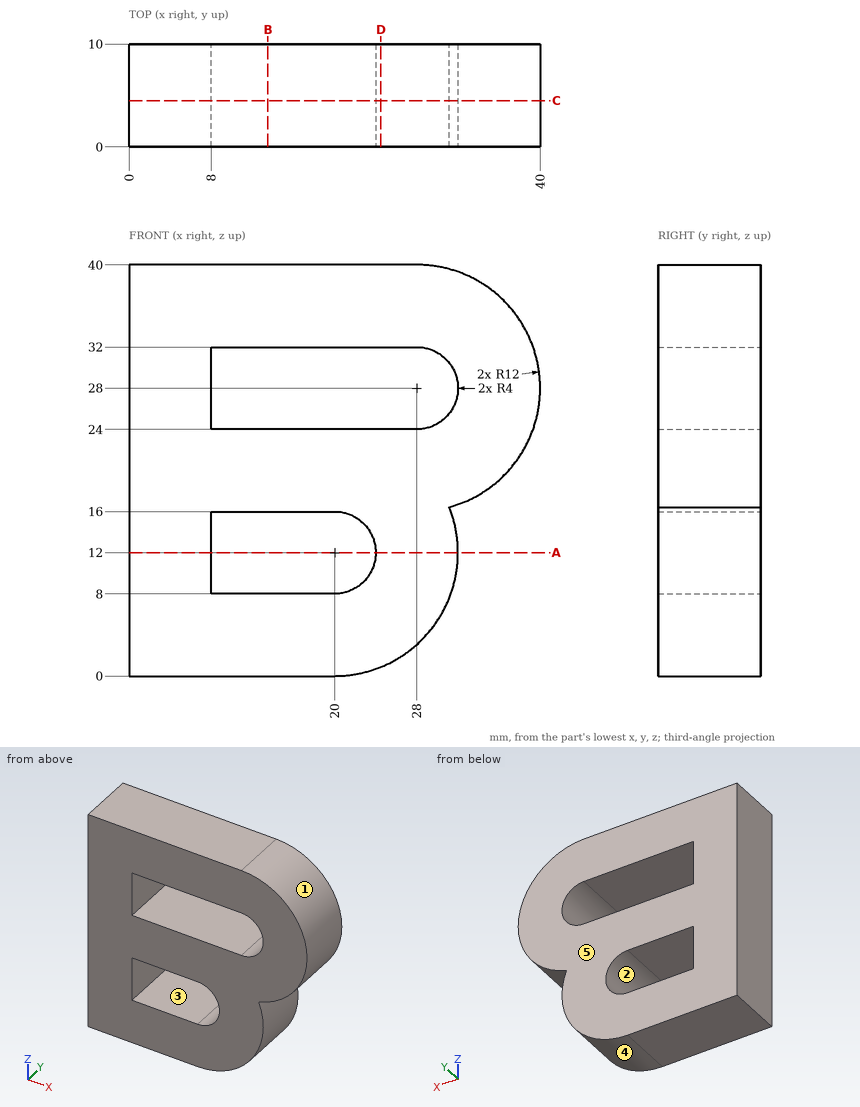
Here's the drawing with two shaded views (mm, measured from the low corner). I have some questions. A direction names the side the tool comes from. Give positions to 0.01 mm unless a question says otherwise; leave off trailing zeros. Write each loop counter-clockwise with the first axis right and the second up, starting at its lowest first coordinate (ties: lowest second). Pieces come first, ordered by that corner, then holes. Notation, with made-up numbers: (87, 60) - (103, 60) arc R27 cw to (103, 85) - close; hole circle Ø5 at (84, -33). An arc over 180 degrees is marked (long way). One line per item, written item: value. Start each with the question number.
Item 1: If we mould it in two halves opening along X, with no side actions, what happens to the marked faces 3, 4 and 5? For each: +X half, -X half, draft (parallel to the pull), parting line (faces both ways), or undercut.
Item 2: Imagine slicing it at C-C, the plane y = 4.5. List the corners of the cut face in (x, z) for me.
Item 3: I'm going to push a flat-ended pin straight in: pin 1 (5 mm diameter, centred on y = 7.5, z = 20.5, fed in from +X). Where does the tip first touch, or does it pass through?
Item 4: Imagine slicing it at A-A, the plane z = 12. List the corners of the cut face in (x, y) for me, and give its area (3 significant figures).
Item 5: Please list where these lines run through material, in increasing order: line 1 (Z direction, x = 17, y = 0.75); line 2 (X direction, y = 7, z = 12.5); line 3 (Z direction, x = 21, y = 8.5). Write a range as from..to.
Item 6: Which directions (+Z, -Z, +X, -X, +Y, -Y) give clear straight access to the entire face, cutting with the end or side of a thin tool? Please do the marked faces 1 and 2.
Item 7: Imagine slicing it at B-B, the plane x = 13.5. List the corners of the cut face in (y, z) for me, and give its area (3 significant figures).
Item 8: Imagine slicing it at D-D, the plane x = 24.5. List the corners of the cut face in (y, z) for me, and give its area (3 significant figures).
Geometry says:
1. face 3: undercut
1. face 4: +X half
1. face 5: draft
2. outline: (0, 0) - (20, 0) arc R12 ccw to (31.16, 16.42) arc R12 ccw to (28, 40) - (0, 40) - close; hole (8, 8) - (20, 8) arc R4 ccw to (20, 16) - (8, 16) - close; hole (8, 24) - (28, 24) arc R4 ccw to (28, 32) - (8, 32) - close
3. pin 1: x = 38.91
4. outline: (0, 0) - (8, 0) - (8, 10) - (0, 10) - close; (24, 0) - (32, 0) - (32, 10) - (24, 10) - close
4. area: 160 mm^2
5. line 1: 0..8, 16..24, 32..40
5. line 2: 0..8, 23.97..31.99
5. line 3: 0.04..8.13, 15.87..24, 32..40
6. face 1: +X, +Y, -Y
6. face 2: +Y, -Y
7. outline: (0, 0) - (10, 0) - (10, 8) - (0, 8) - close; (0, 16) - (10, 16) - (10, 24) - (0, 24) - close; (0, 32) - (10, 32) - (10, 40) - (0, 40) - close
7. area: 240 mm^2
8. outline: (0, 0.88) - (10, 0.88) - (10, 24) - (0, 24) - close; (0, 32) - (10, 32) - (10, 40) - (0, 40) - close
8. area: 311 mm^2
